The listing builds one solid part. Answer for the finished solid, in the listing's coordinates (mm). A direction names the side the tool comes from. Coordinates: 2 decimals unless noted, no trailing zeros. Loops run counter-clockwise (first coordinate to the right, second up) from the corner with the lowest first, then second, coordinate; pieces in that order, holes last. Notation, with made-up numbers: (-33.5, -25.5) - (-8.5, -25.5) arc R23 ccw to (-8.5, 3.5) - close; hole circle Ø6 at (48, 13.25). An arc over 180 degrees is marked (long way). Return JSON: item names as keys, results as strings. Group by question number.
1. Section C-C (x = -29.7) is taken. Write down the section's boundary in (y, z) (3 decimals), and give its area (3 significant figures).
2. The mould has two halves that part along X. Classify faces 4 (the face through (-30.2, 3.04, -2.73)), 5 (the face through (0, 3, -5)), 6 (the face through (-20.553, 7.499, -5.07)), 7 (the face through (-24.8, 6.7, -5.1)): pulls with the +X half, pulls with the -X half, needs draft (parallel to the pull), parting line crosses it, or undercut.
3. Which of the six approach directions +Z, -Z, +X, -X, +Y, -Y give full straight-line access (tool end or side, diameter ignored) to faces 1 (the face through (-4.8, 3.04, -2.73)), 2 (the face through (-24, 9, -5)), 3 (the face through (-3.2, 6, -2.7))?
4. Find the intervals of material crossed by line 1 along X through (y, z) = (2.05, -5) (3 decimals); line 2 along Y through (x, z) = (-17, -4) (3 decimals); line 3 along X through (y, z) = (2.95, -5) (3 decimals), in increasing order.
5. Each of these flat-tipped pins is pushed along its axis until it touches: P1, Ø5.5, axis at x = -29.7, z = -5, coming from the -Y side; P2, Ø4, axis at x = -31, z = -5, coming from the +Y side; P3, Ø0.8, axis at y = 9, z = -6, coming from the -X side; P4, Ø6.5, axis at x = -17, y = 6.38, coming from the -Z side. Where does it stop, or does it pass through?
6. Section D-D (z = -1.5) is taken. Write down the section's boundary in (x, y) (3 decimals), and give its area (3 significant figures).
7. Section B-B (z = -5) is taken. Write down the section's boundary in (x, y) (3 decimals).
8. Section A-A (y = 6.38) is taken. Write down the section's boundary in (x, z) (3 decimals), and give its area (3 significant figures).
Autodesk Inventor part; units mm, degrees
ref_plane "YZ Plane" through (0, 0, 0) normal (1, 0, 0) x (0, 1, 0)
ref_plane "XZ Plane" through (0, 0, 0) normal (0, 1, 0) x (-1, 0, 0)
ref_plane "XY Plane" through (0, 0, 0) normal (0, 0, 1) x (1, 0, 0)
sketch "Sketch1" plane through (0, 0, 0) normal (0, 1, 0) x (-1, 0, 0)
  line L0 (0, 0) -> (34, 0)
  line L1 (34, 0) -> (34, -10)
  line L2 (34, -10) -> (0, -10)
  line L3 (0, -10) -> (0, 0)
  dimension "d0" = 34
  dimension "d1" = 10
extrude "Extrusion1" add sketch "Sketch1" along normal blind 6
sketch "Sketch3" plane through (0, 6, 0) normal (0, 1, 0) x (1, 0, 0)
  circle A0 centre (-4.3, 5) radius 2.325
  line L0 (0, 10) -> (-34, 10)
  circle A1 centre (-29.7, 5) radius 2.325
  line L1 (-34, 10) -> (-34, 0)
  line L2 (0, 0) -> (0, 10)
  dimension "d4" = 4.65
  dimension "d5" = 5
  dimension "d6" = 4.65
  dimension "d7" = 5
  dimension "d9" = 4.3
  dimension "d10" = 4.3
extrude "Extrusion2" cut sketch "Sketch3" against normal through all
sketch "Sketch4" plane through (0, 6, 0) normal (0, 1, 0) x (1, 0, 0)
  line L0 (-34, 0) -> (0, 0)
  line L1 (0, 10) -> (-34, 10)
  line L2 (-10, 0) -> (-24, 0)
  line L3 (-24, 0) -> (-24, 10)
  line L4 (-24, 10) -> (-10, 10)
  line L5 (-10, 10) -> (-10, 0)
  circle A0 centre (-4.3, 5) radius 2.325
  line L6 (-34, 10) -> (-34, 0)
  line L7 (0, 0) -> (0, 10)
  point P0 (-10, 10)
  point P1 (-24, 0)
  dimension "d34" = 14
  dimension "d35" = 10
extrude "Extrusion3" add sketch "Sketch4" along normal blind 8 contours L3 L1 L5 L0
sketch "Sketch6" plane through (0, 0, -10) normal (0, 0, -1) x (-1, 0, 0)
  circle A0 centre (17, 6.38) radius 3.725
  line L0 (10, 14) -> (24, 14)
  line L1 (24, 6) -> (24, 14)
  point P0 (0, 0)
  dimension "d26" = 7.45
  dimension "d36" = 7.62
  dimension "d37" = 7
extrude "Extrusion4" cut sketch "Sketch6" against normal through all
fillet "Fillet2" radius 4 2 edges at (-24, 14, -5) (-10, 14, -5)
chamfer "Chamfer1" distance 1.5 angle 45 2 edges at (-10, 6, -5) (-24, 6, -5)
properties part number "Modular_Single_Axle_V41Y"
The answers:
{
 "1": {"outline": "(0, -10) - (6, -10) - (6, -7.325) - (0, -7.325) - close; (0, -2.675) - (6, -2.675) - (6, 0) - (0, 0) - close", "area": "32.1 mm2"},
 "2": {"face 4": "undercut", "face 5": "pulls with the +X half", "face 6": "undercut", "face 7": "pulls with the -X half"},
 "3": {"face 1": "+Y, -Y", "face 2": "+Z, -Z, -X, +Y", "face 3": "+Z, -Z, +X, +Y"},
 "4": {"line 1": "x = -34 to -32.025, -27.375 to -6.625, -1.975 to 0", "line 2": "y = 0 to 2.655, 10.105 to 14", "line 3": "x = -34 to -32.025, -27.375 to -18.453, -15.547 to -6.625, -1.975 to 0"},
 "5": {"P1": "stops at y = 0", "P2": "stops at y = 6", "P3": "stops at x = -24", "P4": "passes through"},
 "6": {"outline": "(-34, 0) - (0, 0) - (0, 6) - (-8.5, 6) - (-10, 7.5) - (-10, 10) arc R4 ccw to (-14, 14) - (-20, 14) arc R4 ccw to (-24, 10) - (-24, 7.5) - (-25.5, 6) - (-34, 6) - close; hole circle Ø7.45 at (-17, 6.38)", "area": "268 mm2"},
 "7": {"outline": "(-34, 0) - (-32.025, 0) - (-32.025, 6) - (-34, 6) - close; (-27.375, 0) - (-6.625, 0) - (-6.625, 6) - (-8.5, 6) - (-10, 7.5) - (-10, 10) arc R4 ccw to (-14, 14) - (-20, 14) arc R4 ccw to (-24, 10) - (-24, 7.5) - (-25.5, 6) - (-27.375, 6) - close; (-1.975, 0) - (0, 0) - (0, 6) - (-1.975, 6) - close; hole circle Ø7.45 at (-17, 6.38)"},
 "8": {"outline": "(-25.12, -10) - (-20.725, -10) - (-20.725, 0) - (-25.12, 0) - close; (-13.275, -10) - (-8.88, -10) - (-8.88, 0) - (-13.275, 0) - close", "area": "87.9 mm2"}
}
